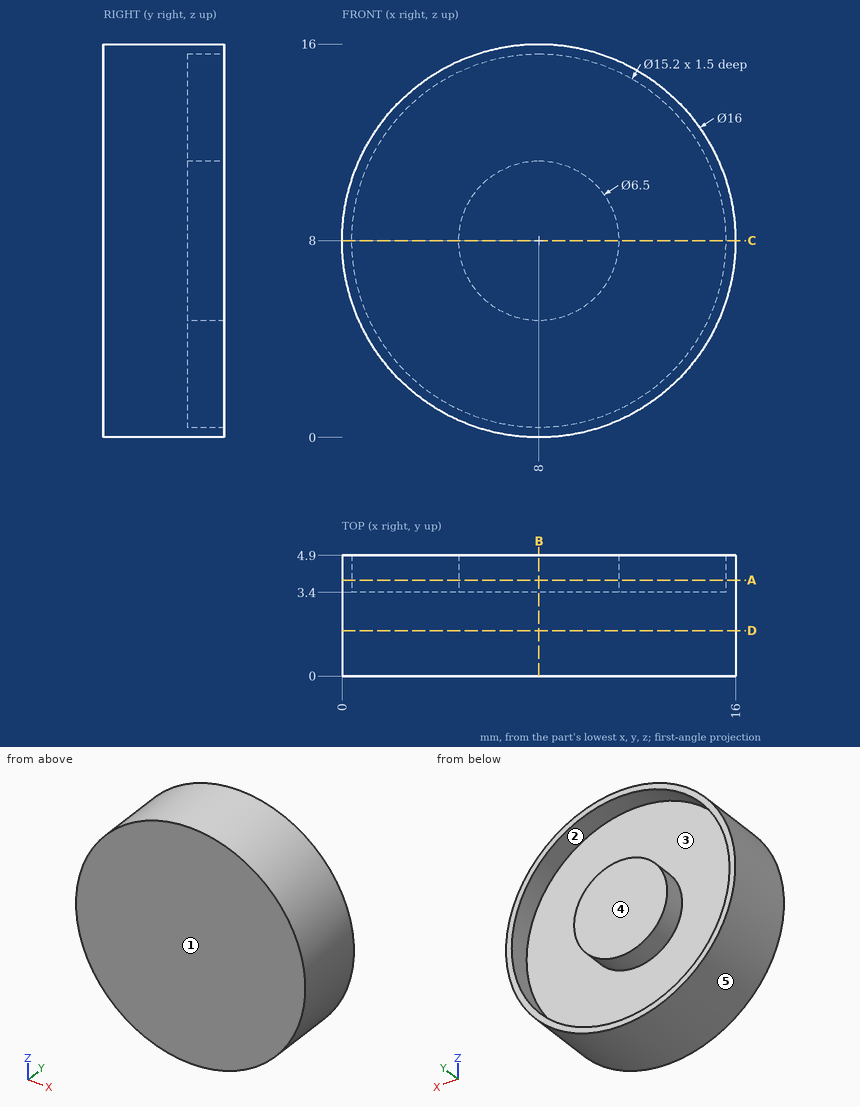
Here's the drawing with two shaded views (mm, measured from the low corner). I have some questions. A direction names the side the tool comes from. Coordinates: 2 decimals unless noted, no trailing zeros. Order: outer loops, then holes, each group sorted by start corner. A loop starts at its lowest first (then second) coordinate and runs counter-clockwise, first axis right, second up. Notation, with made-up numbers: (35, 54.25) - (64, 54.25) arc R16 ccw to (64, 82.25) - close; hole circle Ø11 at (24, 28). An arc over 180 degrees is marked (long way). Answer in a Markdown table with one row per item.
1. If I drill on line 1 along X through (y, z) = (4.2, 8); line 2 along X through (y, z) = (4.5, 9.25); line 3 along Y through (x, z) = (4.5, 13), over which ranges is the centre line in solid material (lowest first)?
Reply:
| item | result |
|---|---|
| line 1 | x = 0 to 0.4, 4.75 to 11.25, 15.6 to 16 |
| line 2 | x = 0.1 to 0.5, 5 to 11, 15.5 to 15.9 |
| line 3 | y = 0 to 3.4 |
2. Suppose I cut it at B-B (x = 8). Please give me the cut outline in (y, z).
Reply:
| item | result |
|---|---|
| outline | (0, 0) - (4.9, 0) - (4.9, 0.4) - (3.4, 0.4) - (3.4, 4.75) - (4.9, 4.75) - (4.9, 11.25) - (3.4, 11.25) - (3.4, 15.6) - (4.9, 15.6) - (4.9, 16) - (0, 16) - close |
3. Suppose I cut it at C-C (z = 8). Please give me the cut outline in (x, y), and give its area (4 significant figures).
Reply:
| item | result |
|---|---|
| outline | (0, 0) - (16, 0) - (16, 4.9) - (15.6, 4.9) - (15.6, 3.4) - (11.25, 3.4) - (11.25, 4.9) - (4.75, 4.9) - (4.75, 3.4) - (0.4, 3.4) - (0.4, 4.9) - (0, 4.9) - close |
| area | 65.35 mm^2 |
4. If we mould it in two halves opening along X, with no side actions, what happens to the marked faces 3, 4 and 5? For each: pulls with the +X half, pulls with the -X half, needs draft (parallel to the pull), parting line crosses it, or undercut.
Reply:
| item | result |
|---|---|
| face 3 | undercut |
| face 4 | needs draft |
| face 5 | parting line crosses it |
5. For the marked faces 1 and 2, which set-ups out of +Z, -Z, +X, -X, +Y, -Y let a thin tool reach every point of the face, with its end or its side?
Reply:
| item | result |
|---|---|
| face 1 | +Z, -Z, +X, -X, -Y |
| face 2 | +Y |
6. Suppose I cut it at A-A (y = 3.9). Please give me the cut outline in (x, z).
Reply:
| item | result |
|---|---|
| outline | circle Ø16 at (8, 8); circle Ø6.5 at (8, 8); hole circle Ø15.2 at (8, 8) |
7. Suppose I cut it at D-D (y = 1.85). Please give me the cut outline in (x, z), and give its area (3 significant figures).
Reply:
| item | result |
|---|---|
| outline | circle Ø16 at (8, 8) |
| area | 201 mm^2 |
